Geometry check sheet. Reference: the model listing, model coordinates, mm. Face numbers are marked on the shaded views. A direction names the side the tool comes from. Coordinates: 2 decimals unless noted, no trailing zeros. Order: outer loops, then holes, each group sorted by start corner. A loop starts at its lowest first (then second) coordinate and runs counter-clockwise, first axis right, second up. Notation, with made-up numbers: M 4,-26.5 L 59,-26.5 A18 cw 59,-10.5 Z; hole C 17.5,-27 d5. An arc over 180 degrees is marked long. Use CSV: the item, a comma, the result in double quotes. Start each with the question number.
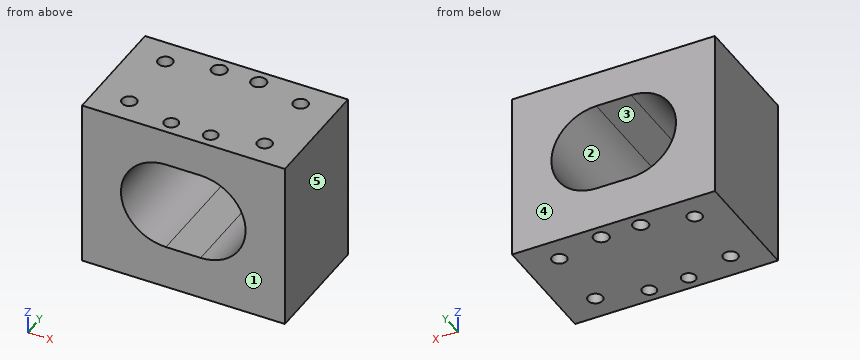
```python
from build123d import *

# Parameters (mm, degrees)
SKETCH_1_W          = 36
SKETCH_1_H          = 21
SKETCH_1_R          = 1.25
SKETCH_1_R_2        = 1.3
SKETCH_1_R_3        = 1.35
EXTRUDE_1_DEPTH     = 30
SKETCH_1_5_R        = 1.3
SKETCH_1_5_R_2      = 1.35
SKETCH_1_5_R_3      = 1.25
CUT_EXTRUDE_1_DEPTH = 4
CUT_EXTRUDE_START   = 30
SKETCH_1_6_R        = 1.35
SKETCH_1_6_R_2      = 1.3
SKETCH_1_6_R_3      = 1.25
CUT_EXTRUDE_2_DEPTH = 4
CUT_EXTRUDE1_DEPTH  = 30


with BuildPart() as part:
    # 스케치1 → 보스-돌출1 (new body)
    with BuildSketch(Plane.XY):
        Rectangle(SKETCH_1_W, SKETCH_1_H)
        with Locations((-3.5, -8)):
            Circle(SKETCH_1_R, mode=Mode.SUBTRACT)
        with Locations((3.5, -8)):
            Circle(SKETCH_1_R, mode=Mode.SUBTRACT)
        with Locations((-12, 6)):
            Circle(SKETCH_1_R_2, mode=Mode.SUBTRACT)
        with Locations((12, 6)):
            Circle(SKETCH_1_R_2, mode=Mode.SUBTRACT)
        with Locations((12, -6)):
            Circle(SKETCH_1_R_2, mode=Mode.SUBTRACT)
        with Locations((-12, -6)):
            Circle(SKETCH_1_R_2, mode=Mode.SUBTRACT)
        with Locations((3.5, 8)):
            Circle(SKETCH_1_R_3, mode=Mode.SUBTRACT)
        with Locations((-3.5, 8)):
            Circle(SKETCH_1_R_3, mode=Mode.SUBTRACT)
        with Locations((12, -6)):
            Circle(SKETCH_1_R_2)
        with Locations((3.5, -8)):
            Circle(SKETCH_1_R)
        with Locations((-3.5, -8)):
            Circle(SKETCH_1_R)
        with Locations((-12, -6)):
            Circle(SKETCH_1_R_2)
        with Locations((-12, 6)):
            Circle(SKETCH_1_R_2)
        with Locations((-3.5, 8)):
            Circle(SKETCH_1_R_3)
        with Locations((3.5, 8)):
            Circle(SKETCH_1_R_3)
        with Locations((12, 6)):
            Circle(SKETCH_1_R_2)
    extrude(amount=EXTRUDE_1_DEPTH)

    # 스케치1<5> → 컷-돌출1 (cut)
    with BuildSketch(Plane.XY):
        with Locations((12, 6)):
            Circle(SKETCH_1_5_R)
        with Locations((3.5, 8)):
            Circle(SKETCH_1_5_R_2)
        with Locations((-3.5, 8)):
            Circle(SKETCH_1_5_R_2)
        with Locations((-12, 6)):
            Circle(SKETCH_1_5_R)
        with Locations((-12, -6)):
            Circle(SKETCH_1_5_R)
        with Locations(Location((-3.5, -8, 0), (0, 0, 180))):
            Circle(SKETCH_1_5_R_3)
        with Locations((3.5, -8)):
            Circle(SKETCH_1_5_R_3)
        with Locations((12, -6)):
            Circle(SKETCH_1_5_R)
    extrude(amount=CUT_EXTRUDE_1_DEPTH, mode=Mode.SUBTRACT)

    # 스케치1<6> → 컷-돌출2 (cut)
    with BuildSketch(Plane.XY.offset(CUT_EXTRUDE_START)):
        with Locations((3.5, 8)):
            Circle(SKETCH_1_6_R)
        with Locations((12, 6)):
            Circle(SKETCH_1_6_R_2)
        with Locations((-3.5, 8)):
            Circle(SKETCH_1_6_R)
        with Locations((-12, 6)):
            Circle(SKETCH_1_6_R_2)
        with Locations((-12, -6)):
            Circle(SKETCH_1_6_R_2)
        with Locations(Location((-3.5, -8, 0), (0, 0, 180))):
            Circle(SKETCH_1_6_R_3)
        with Locations((3.5, -8)):
            Circle(SKETCH_1_6_R_3)
        with Locations((12, -6)):
            Circle(SKETCH_1_6_R_2)
    extrude(amount=-CUT_EXTRUDE_2_DEPTH, mode=Mode.SUBTRACT)

    # Sketch1 → Cut-Extrude1 (cut)
    with BuildSketch(Plane(origin=(0, 10.5, 0), x_dir=(1, 0, 0), z_dir=(0, 1, 0))):
        with BuildLine():
            Line((-3.118018925, -7.687381661), (3.044704105, -7.687381661))
            ThreePointArc((3.044704105, -7.687381661), (11.019992732, -15.662670288), (3.044704105, -23.637958915))
            Line((3.044704105, -23.637958915), (-3.118018925, -23.637958915))
            ThreePointArc((-3.118018925, -23.637958915), (-11.093307551, -15.662670288), (-3.118018925, -7.687381661))
        make_face()
    extrude(amount=-CUT_EXTRUDE1_DEPTH, mode=Mode.SUBTRACT)


solid = part.part
```
1) Gauge pin test, flat ends, axial feed: P1, Ø2, axis at x = -12, y = -6, coming from the +Z side; P2, Ø1.3, axis at x = 11.5, y = -6, coming from the -Z side. Record the tip position at first contact, or that the pin passes through.
2) Section check D-D on x = -12. Record the boundary of the cut face in (y, z), then the cut area to 3 significant figures.
3) Draft check along X on the marked faces 3, 4 and 5. Enter one of: +X half, -X half, draft (parallel to the pull), parting line (faces both ways), or undercut.
4) Material ranges on line 1 along Y through (x, z) = (3.5, 27.8); line 2 along Y through (x, z) = (12, 27); line 3 along X through (y, z) = (-5, 15.5), recorded low to high.
5) Section check A-A on x = 0. Record the boundary of the cut face in (y, z).
6) Section check B-B on z = 13.5. Record the boundary of the cut face in (x, y).
7) Set-up check for the marked faces 1 and 2: record each of +Z, -Z, +X, -X, +Y, -Y from which the full face is reachable in a straight line by a thin tool's end or side.
Results are:
1,P1,"stops at z = 26"
1,P2,"stops at z = 4"
2,outline,"M -10.5,0 L -7.3,0 L -7.3,4 L -4.7,4 L -4.7,0 L 4.7,0 L 4.7,4 L 7.3,4 L 7.3,0 L 10.5,0 L 10.5,30 L 7.3,30 L 7.3,26 L 4.7,26 L 4.7,30 L -4.7,30 L -4.7,26 L -7.3,26 L -7.3,30 L -10.5,30 Z"
2,area,"588 mm²"
3,face 3,"undercut"
3,face 4,"draft"
3,face 5,"+X half"
4,line 1,"y = -10.5 to -9.25, -6.75 to 6.65, 9.35 to 10.5"
4,line 2,"y = -10.5 to -7.3, -4.7 to 4.7, 7.3 to 10.5"
4,line 3,"x = -18 to -11.09, 11.02 to 18"
5,outline,"M -10.5,0 L 10.5,0 L 10.5,7.69 L -10.5,7.69 Z; M -10.5,23.64 L 10.5,23.64 L 10.5,30 L -10.5,30 Z"
6,outline,"M -18,-10.5 L -10.79,-10.5 L -10.79,10.5 L -18,10.5 Z; M 10.72,-10.5 L 18,-10.5 L 18,10.5 L 10.72,10.5 Z"
7,face 1,"+Z, -Z, +X, -X, -Y"
7,face 2,"+Y, -Y"
